Input: part model. Units: mm. Frame: model coordinates. Face numbers are marked on the shaded views. A direction names the side the tool comes from. Coordinates: 2 decimals unless noted, no trailing zeros. Order: outer loops, then holes, each group sorted by start corner. A loop starts at its lowest first (then second) coordinate and runs counter-clockwise, first axis right, second up. Notation, with made-up numbers: M -37.5,-3 L -3.5,-3 A6 ccw -3.5,8 Z; hole C 25.5,5 d2. An arc over 180 degrees is marked long. One line per item, written item: value.
Autodesk Fusion 360 part; units mm, degrees
sketch "Sketch1" plane through (0, 0, 0) normal (0, 0, 1) x (1, 0, 0)
  line L0 (4.8, -5) -> (-4.8, -5)
  line L1 (-4.8, -5) -> (-4.8, 5)
  line L2 (4.8, 5) -> (4.8, -5)
  line L3 (4.8, -5) -> (-4.8, 5) construction
  line L4 (-4.8, -5) -> (4.8, 5) construction
  line L5 (-4.8, -5) -> (4.8, -5)
  line L6 (4.8, -7.5) -> (4.8, -45)
  line L7 (4.8, -45) -> (-4.8, -45)
  line L8 (-4.8, -45) -> (-4.8, -7.5)
  line L9 (-10.3, -7.5) -> (-10.3, 7.5)
  line L10 (10.3, 7.5) -> (10.3, -7.5)
  line L11 (10.3, -7.5) -> (-10.3, 7.5) construction
  line L12 (-10.3, -7.5) -> (10.3, 7.5) construction
  line L13 (4.8, 5) -> (10.3, 5)
  line L14 (-4.8, 5) -> (-10.3, 5)
  line L15 (10.3, -7.5) -> (4.8, -7.5)
  line L16 (-4.8, -7.5) -> (-10.3, -7.5)
  dimension "d1" = 9.6
  dimension "d3" = 9.6
  dimension "d4" = 40
  dimension "d5" = 20.6
extrude "Extrude1" add sketch "Sketch1" along normal blind 10
fillet "Fillet1" radius 3.5 2 edges at (0, -45, 10) (0, -45, 0)
chamfer "Chamfer1" distance 4 angle 45 2 edges at (-4.8, -7.5, 5) (4.8, -7.5, 5)
fillet "Fillet2" radius 4.5 2 edges at (10.3, 5, 5) (-10.3, 5, 5)
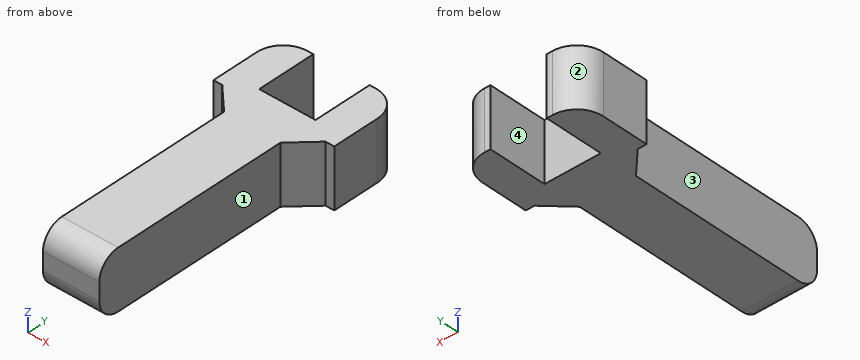
(1) Ray query, line 1 (X direction, y = 0, z = 8.5); line 2 (X direction, y = -31, z = 1); line 3 (X direction, y = -10.5, z = 6.5). Return the intervals inside material, ascending. Write a range as from..to.
Data:
line 1: x = -10.3..-4.8, 4.8..10.3
line 2: x = -4.8..4.8
line 3: x = -5.8..5.8
(2) First-contact query: pin 1 (0.8 mm diameter, centred on x = -9.5, z = 7, fed in from -Y); pin 2 (3 mm diameter, centred on y = -20.5, z = 5, fed in from +X). Flat tips, straight axial feed; report the tip coordinate or a pass-through.
Data:
pin 1: stops at y = -7.5
pin 2: stops at x = 4.8
(3) Cut plane C-C on z = 4. Output: boundary loops of the cut face in (x, y).
Data:
outline: M -10.3,-7.5 L -8.8,-7.5 L -4.8,-11.5 L -4.8,-45 L 4.8,-45 L 4.8,-11.5 L 8.8,-7.5 L 10.3,-7.5 L 10.3,0.5 A4.5 ccw 5.8,5 L 4.8,5 L 4.8,-5 L -4.8,-5 L -4.8,5 L -5.8,5 A4.5 ccw -10.3,0.5 Z
(4) Cut plane A-A on y = -4. Output: boundary loops of the cut face in (x, z).
Data:
outline: M -10.3,0 L -4.8,0 L -4.8,10 L -10.3,10 Z; M 4.8,0 L 10.3,0 L 10.3,10 L 4.8,10 Z
(5) Cut plane D-D on y = -14.5. Output: boundary loops of the cut face in (x, z).
Data:
outline: M -4.8,0 L 4.8,0 L 4.8,10 L -4.8,10 Z
(6) Access query for the marked faces 1, 2, 3 and 4. Directions: +Z, -Z, +X, -X, +Y, -Y. A direction counts if a zero-diameter tool reaches every point of the face in a straight line with its end or side. Return the directions, or none.
Data:
face 1: +Z, -Z, +X, -Y
face 2: +Z, -Z, -X, +Y
face 3: +Z, -Z, -X, -Y
face 4: +Z, -Z, +Y
(7) Cut plane B-B on x = 2.25. Output: boundary loops of the cut face in (y, z).
Data:
outline: M -45,3.5 A3.5 ccw -41.5,0 L -5,0 L -5,10 L -41.5,10 A3.5 ccw -45,6.5 Z
